Source: three-view drawing plus pictorial views. Frame: mm from the lowest corner of the part. A direction names the side the tool comes from. Give positions to 0.01 mm unless a question says otherwise; leave off trailing zeros. Loops run counter-clockwise (first coordinate to the right, second up) from the corner with the lowest first, then second, coordinate; pieces in that order, holes last. Notation, with made-up numbers: (-16, -29.75) - (24, -29.75) arc R10 cw to (24, -14.75) - close; hole circle Ø1 at (68, -29.5). An arc over 180 degrees is marked (long way). Answer as a JSON object with one key per item and string values.
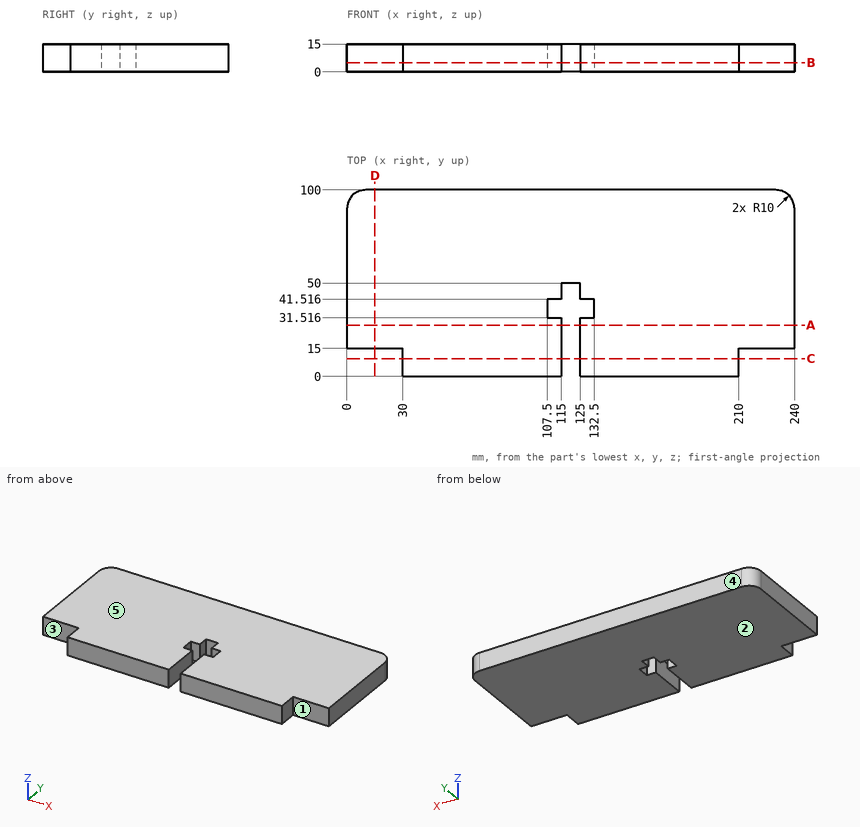
Item 1: Cut plane B-B (z = 5). Return loops of the section in (x, y).
Geometry check:
{"outline": "(0, 15) - (30, 15) - (30, 0) - (115, 0) - (115, 31.52) - (107.5, 31.52) - (107.5, 41.52) - (115, 41.52) - (115, 50) - (125, 50) - (125, 41.52) - (132.5, 41.52) - (132.5, 31.52) - (125, 31.52) - (125, 0) - (210, 0) - (210, 15) - (240, 15) - (240, 90) arc R10 ccw to (230, 100) - (10, 100) arc R10 ccw to (0, 90) - close"}
Item 2: Access query for the marked faces 1 and 2. Directions: +Z, -Z, +X, -X, +Y, -Y. A direction counts if a zero-diameter tool reaches every point of the face in a straight line with its end or side. Return the directions, or none.
Geometry check:
{"face 1": "+Z, -Z, +X, -Y", "face 2": "-Z, +X, -X, +Y, -Y"}
Item 3: Cut plane C-C (y = 9.5). Return loops of the section in (x, z).
Geometry check:
{"outline": "(30, 0) - (115, 0) - (115, 15) - (30, 15) - close; (125, 0) - (210, 0) - (210, 15) - (125, 15) - close"}
Item 4: Cut plane A-A (y = 27.5). Return loops of the section in (x, z).
Geometry check:
{"outline": "(0, 0) - (115, 0) - (115, 15) - (0, 15) - close; (125, 0) - (240, 0) - (240, 15) - (125, 15) - close"}
Item 5: Cut plane D-D (x = 15). Return loops of the section in (y, z).
Geometry check:
{"outline": "(15, 0) - (100, 0) - (100, 15) - (15, 15) - close"}
Item 6: Contact query for flat-ended pins moving along their axis: P1, Ø7.5, axis at y = 9, z = 11, coming from the +X side; P2, Ø7.5, axis at x = 8.5, z = 5, coming from the -Y side; P3, Ø5, axis at x = 118.5, z = 9.5, coming from the -Y side. Output: stop coordinate, or through.
Geometry check:
{"P1": "stops at x = 210", "P2": "stops at y = 15", "P3": "stops at y = 50"}
Item 7: Mould query, pull axis Y, two halves, no side actions, for the marked faces 3, 4 and 5. Classes: released by +Y, released by -Y, zero draft, split by the parting line, or undercut.
Geometry check:
{"face 3": "released by -Y", "face 4": "released by +Y", "face 5": "zero draft"}
Item 8: Material intervals for line 1 (X direction, y = 49.5, z = 11); line 2 (Y direction, x = 129.5, z = 8.75); line 3 (Y direction, x = 27, z = 13), sorted ascending. Write a range as [from, to].
Geometry check:
{"line 1": "x = [0, 115], [125, 240]", "line 2": "y = [0, 31.52], [41.52, 100]", "line 3": "y = [15, 100]"}
